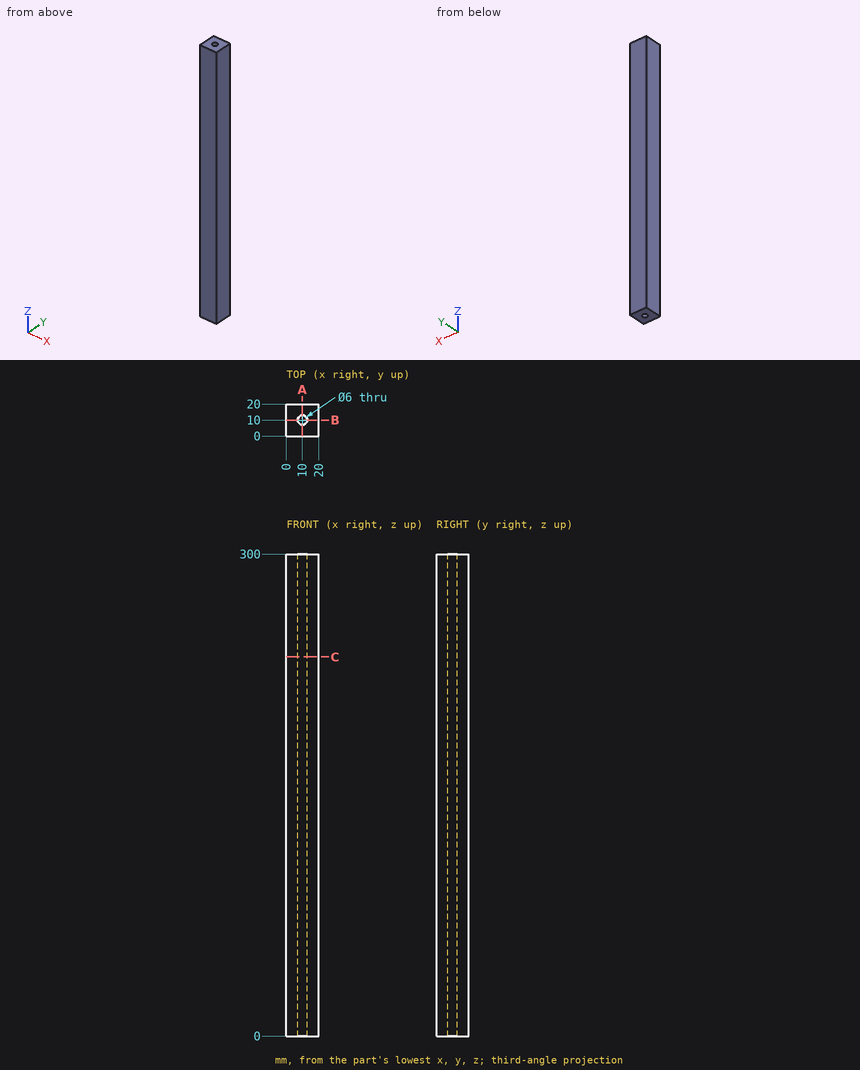
Source: three-view drawing plus pictorial views. Frame: mm from the lowest corner of the part. Give positions to 0.01 mm unless a question says otherwise; leave off trailing zeros. Write each loop counter-clockwise with the first axis right and the second up, starting at its lowest first coordinate (ties: lowest second). Pieces come first, ordered by that corner, then holes. Notation, with made-up numbers: (71.25, 51.5) - (107.25, 51.5) arc R24 cw to (107.25, 73.5) - close; hole circle Ø9 at (83.25, 36.5). An arc over 180 degrees is marked (long way). Write item = value, one per line. Start each with the question number.
Q1. Cut plane A-A, the plane x = 10. Return loops of the section in (y, z), then the cut area to 3 significant figures.
Q2. Material intervals for probe 1 along X at (y, z) = (10, 161.5); probe 2 along Y at (x, z) = (8.5, 105), sorted ascending.
Q3. Pin query (flat end, axial travel): pin 1 Ø3.5 at (x, y) = (10, 10) entering from -Z. Return the tip coordinate at first contact, or that it passes through.
Q4. Cut plane C-C, the plane z = 236. Return loops of the section in (x, y), then the cut area to 3 significant figures.
Computed values:
q1.outline = (0, 0) - (7, 0) - (7, 300) - (0, 300) - close; (13, 0) - (20, 0) - (20, 300) - (13, 300) - close
q1.area = 4,200 mm²
q2.probe_1 = 0 to 7, 13 to 20
q2.probe_2 = 0 to 7.4, 12.6 to 20
q3.pin_1 = through
q4.outline = (0, 0) - (20, 0) - (20, 20) - (0, 20) - close; hole circle Ø6 at (10, 10)
q4.area = 372 mm²
